```python
from build123d import *

# Parameters (mm, degrees)
F0_W     = 139.7
F0_H     = 38.1
F1_DEPTH = 2057.4
F2_W     = 19.05
F2_H     = 38.1
F3_DEPTH = 139.7
F5_DEPTH = 6.35
F7_DEPTH = 6.35


with BuildPart() as f1:
    # F0 (on Top) → F1 (new body)
    with BuildSketch(Plane.XY):
        Rectangle(F0_W, F0_H)
    extrude(amount=F1_DEPTH)

    # F2 (on face) → F3 (cut)
    with BuildSketch(Plane.YZ.offset(69.85)):
        with Locations((-9.525, 698.5)):
            Rectangle(F2_W, F2_H)
        with Locations((-9.525, 1358.9)):
            Rectangle(F2_W, F2_H)
    extrude(amount=-F3_DEPTH, mode=Mode.SUBTRACT)

    # F4 (on face) → F5 (cut)
    with BuildSketch(Plane.XZ.offset(19.05)):
        with BuildLine():
            ThreePointArc((-3.175, 2042.8458), (0, 2039.6708), (3.175, 2042.8458))
            Line((3.175, 2042.8458), (-3.175, 2042.8458))
        make_face()
        with BuildLine():
            Line((-3.175, 2042.8458), (3.175, 2042.8458))
            ThreePointArc((3.175, 2042.8458), (0, 2046.0208), (-3.175, 2042.8458))
        make_face()
    extrude(amount=-F5_DEPTH, mode=Mode.SUBTRACT)

    # F6 (on face) → F7 (cut)
    with BuildSketch(Plane.XZ.offset(19.05)):
        with BuildLine():
            ThreePointArc((-3.175, 14.5542), (0, 11.3792), (3.175, 14.5542))
            Line((3.175, 14.5542), (-3.175, 14.5542))
        make_face()
        with BuildLine():
            Line((-3.175, 14.5542), (3.175, 14.5542))
            ThreePointArc((3.175, 14.5542), (0, 17.7292), (-3.175, 14.5542))
        make_face()
    extrude(amount=-F7_DEPTH, mode=Mode.SUBTRACT)


solid = f1.part
```
The model under review builds one solid part; all positions refer to its coordinate system, in mm. A direction names the side the tool comes from. Coordinates: 2 decimals unless noted, no trailing zeros. Order: outer loops, then holes, each group sorted by start corner. A loop starts at its lowest first (then second) coordinate and runs counter-clockwise, first axis right, second up. Notation, with made-up numbers: (-1, -1.5) -> (46, -1.5) arc R13 cw to (46, 5.5) -> close; hole circle Ø6 at (-8.75, 35.5). An arc over 180 degrees is marked (long way). Answer in a Markdown table with one row per item. Add a question column.
Item 1: We need section A-A on x = -49.5. Write out the cut boundary in (y, z).
Item 2: To check wall thickness, follow probe 1 along Z at (x, y) = (-9.5, -16); probe 2 along Z at (x, y) = (0, -15). State the ranges of each line that lie inside material, in increasing order.
Item 3: Machinability: for faces 1 (the flat face through (1, 0, 1359)), 2 (the flat face through (-1, -19.05, 1713)), which of the approach directions +Z, -Z, +X, -X, +Y, -Y give a long, thin tool a straight path to every point of the face, cutting with its end or side? Answer none if there is none.
Item 4: Mouldability with a two-part tool opening along Z and no side actions: class faces 3 (the flat face through (-1, 0, 2057.4)), 4 (the flat face through (-1, 0, 0)), 5 (the flat face through (1, 0, 698)), 6 (the flat face through (-1, -19.05, 1024)) as +Z half, -Z half, draft (parallel to the pull), parting line (faces both ways), or undercut.
Item 5: Clearance check with flat-ended pins moving along their axes: pin 1 (5.5 mm diameter, centred on x = -20.5, y = -10, fed in from -Z); pin 2 (3 mm diameter, centred on x = 0, z = 13.5, fed in from -Y). State where each tip first meets the part, or that it passes through.
Final values:
| question | item | result |
|---|---|---|
| 1 | outline | (-19.05, 0) -> (19.05, 0) -> (19.05, 2057.4) -> (-19.05, 2057.4) -> (-19.05, 1377.95) -> (0, 1377.95) -> (0, 1339.85) -> (-19.05, 1339.85) -> (-19.05, 717.55) -> (0, 717.55) -> (0, 679.45) -> (-19.05, 679.45) -> close |
| 2 | probe 1 | z = 0 to 679.45, 717.55 to 1339.85, 1377.95 to 2057.4 |
| 2 | probe 2 | z = 0 to 11.38, 17.73 to 679.45, 717.55 to 1339.85, 1377.95 to 2039.67, 2046.02 to 2057.4 |
| 3 | face 1 | +X, -X, -Y |
| 3 | face 2 | +Z, -Z, +X, -X, -Y |
| 4 | face 3 | +Z half |
| 4 | face 4 | -Z half |
| 4 | face 5 | undercut |
| 4 | face 6 | draft |
| 5 | pin 1 | stops at z = 0 |
| 5 | pin 2 | stops at y = -12.7 |
